Could you check a few things on this model? Use its own coordinates, in mm. Face numbers are marked on the shaded views. A direction names the side the tool comes from. Coordinates: 2 decimals unless noted, no trailing zeros. Order: outer loops, then holes, each group sorted by start corner. A loop starts at its lowest first (then second) coordinate and runs counter-clockwise, first axis right, second up. Notation, with made-up numbers: (14, 52.25) - (70, 52.25) arc R30 cw to (70, 76.25) - close; hole circle Ø2 at (77, -12). An arc over 180 degrees is marked (long way). Answer as a JSON object with one key per item and string values. Group by question number.
(1) Imagine slicing it at D-D, the plane x = 0. Write out the boundary of the cut face in (y, z).
(2) Please list where these lines run through material, in increasing order: probe 1 along Y at (x, z) = (0.75, -2); probe 2 along X at (y, z) = (-3.5, 0); probe 3 along Y at (x, z) = (9, 1.5).
(3) Which directions (+Z, -Z, +X, -X, +Y, -Y) give clear straight access to the entire face, cutting with the end or side of a thin tool? Please do the marked faces 1 and 2.
(4) Imagine slicing it at B-B, the plane x = -2.75. Write out the boundary of the cut face in (y, z).
(5) Imagine slicing it at A-A, the plane y = 1. Write out the boundary of the cut face in (x, z).
(6) Imagine slicing it at C-C, the plane z = -0.25. Write out the boundary of the cut face in (x, y).
(7) Will these pins go through, and if not, where does the flat tip stop? P1, Ø4, axis at y = -3.5, z = 2, coming from the +X side; P2, Ø2, axis at y = -2, z = 3, coming from the +X side; P3, Ø1.4, axis at x = 0, z = 0, coming from the +Y side.
(8) We'd pull the mould along Z, two halves only. Please class the marked faces 3, 4 and 5: pulls with the +Z half, pulls with the -Z half, needs draft (parallel to the pull), parting line crosses it, or undercut.
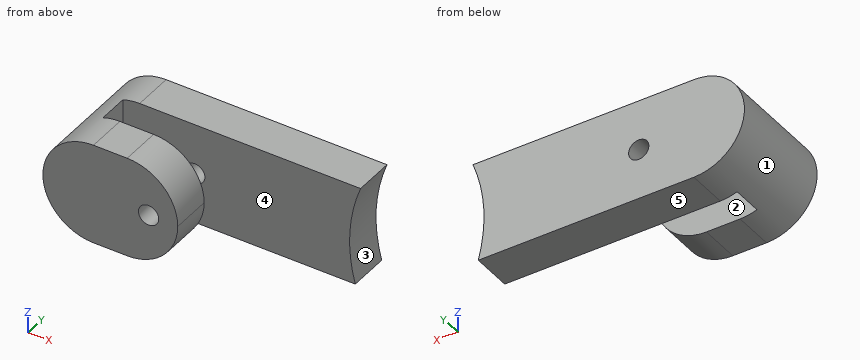
from build123d import *

# Parameters (mm, degrees)
SKETCH1_W           = 18.396209947
SKETCH1_H           = 7.5
BOSS_EXTRUDE1_DEPTH = 3
SKETCH3_W           = 7.837448939
SKETCH3_H           = 7.5
BOSS_EXTRUDE2_DEPTH = 3
SKETCH4_R           = 12
CUT_EXTRUDE2_DEPTH  = 3
SKETCH6_W           = 2.5
SKETCH6_H           = 7.5
BOSS_EXTRUDE3_DEPTH = 5.25
SKETCH7_W           = 7.5
SKETCH7_H           = 3
BOSS_EXTRUDE4_DEPTH = 7.5
CUT_EXTRUDE1_REACH  = 17.271
SKETCH2_R           = 0.75
FILLET1_R           = 3.75


with BuildPart() as part:
    # Sketch1 → Boss-Extrude1 (new body)
    with BuildSketch(Plane(origin=(0, 0, 0), x_dir=(1, 0, 0), z_dir=(0, 1, 0))):
        with Locations((9.198104974, 0)):
            Rectangle(SKETCH1_W, SKETCH1_H)
    extrude(amount=BOSS_EXTRUDE1_DEPTH)

    # Sketch3 → Boss-Extrude2 (add)
    with BuildSketch(Plane(origin=(0, 3, 0), x_dir=(1, 0, 0), z_dir=(0, 1, 0))):
        with Locations((-3.91872447, 0)):
            Rectangle(SKETCH3_W, SKETCH3_H)
    extrude(amount=-BOSS_EXTRUDE2_DEPTH)

    # Sketch4 → Cut-Extrude2 (cut)
    with BuildSketch(Plane(origin=(0, 3, 0), x_dir=(1, 0, 0), z_dir=(0, 1, 0))):
        with Locations((23.476391496, 0.596984019)):
            Circle(SKETCH4_R)
    extrude(amount=-CUT_EXTRUDE2_DEPTH, mode=Mode.SUBTRACT)

    # Sketch6 → Boss-Extrude3 (add)
    with BuildSketch(Plane.XZ):
        with Locations((-6.587448939, 0)):
            Rectangle(SKETCH6_W, SKETCH6_H)
    extrude(amount=BOSS_EXTRUDE3_DEPTH)

    # Sketch7 → Boss-Extrude4 (add)
    with BuildSketch(Plane(origin=(-5.337448939, 0, 0), x_dir=(0, 0, -1), z_dir=(1, 0, 0))):
        with Locations((0, -3.75)):
            Rectangle(SKETCH7_W, SKETCH7_H)
    extrude(amount=BOSS_EXTRUDE4_DEPTH)

    # Cut-Extrude1: up to this face of the body (flat: up to its plane)
    cut_extrude1_end = Plane(part.part.faces().sort_by_distance((-2.837448939, -5.25, 0))[0])
    # Sketch2 → Cut-Extrude1 (cut, up to the picked face)
    with BuildSketch(Plane(origin=(0, 3, 0), x_dir=(1, 0, 0), z_dir=(0, 1, 0)), mode=Mode.PRIVATE) as cut_extrude1_sk1:
        with Locations(Location((0, 0, 0), (0, 0, 90))):
            Circle(SKETCH2_R)
    cut_extrude1_tool1 = split(extrude(cut_extrude1_sk1.sketch, amount=-CUT_EXTRUDE1_REACH, mode=Mode.PRIVATE), bisect_by=cut_extrude1_end, keep=Keep.BOTH, mode=Mode.PRIVATE)
    add(cut_extrude1_tool1.solids().sort_by(Axis((0, 3, 0), (0, -1, 0)))[0], mode=Mode.SUBTRACT)

    # Fillet1
    # the kernel refuses this fillet: 3.75 mm, written as the material it takes off along each edge
    with BuildSketch(Plane(origin=(2.162551061, -14.625, -3.75), x_dir=(0, 0, 1), z_dir=(0, 1, 0))) as fillet1_piece_1:
        with BuildLine():
            CenterArc((FILLET1_R, -FILLET1_R), FILLET1_R, 90, 90)
            Line((0, -FILLET1_R), (0, 0))
            Line((0, 0), (FILLET1_R, 0))
        make_face()
    extrude(amount=12.375, mode=Mode.SUBTRACT)
    with BuildSketch(Plane(origin=(2.162551061, -2.25, 3.75), x_dir=(-1, 0, 0), z_dir=(0, -1, 0))) as fillet1_piece_2:
        with BuildLine():
            CenterArc((FILLET1_R, FILLET1_R), FILLET1_R, 180, 90)
            Line((0, FILLET1_R), (0, 0))
            Line((0, 0), (FILLET1_R, 0))
        make_face()
    extrude(amount=12.375, mode=Mode.SUBTRACT)
    with BuildSketch(Plane(origin=(-7.837448939, 12.375, 3.75), x_dir=(1, 0, 0), z_dir=(0, -1, 0)), Plane(origin=(-7.837448939, 12.375, -3.75), x_dir=(0, 0, 1), z_dir=(0, -1, 0))) as fillet1_piece_3:
        with BuildLine():
            CenterArc((FILLET1_R, -FILLET1_R), FILLET1_R, 90, 90)
            Line((0, -FILLET1_R), (0, 0))
            Line((0, 0), (FILLET1_R, 0))
        make_face()
    extrude(amount=27, mode=Mode.SUBTRACT)


solid = part.part
Result set:
{
 "1": {"outline": "(-5.25, -3.4) - (-2.25, -3.4) - (-2.25, -0.75) - (-5.25, -0.75) - close; (-5.25, 0.75) - (-2.25, 0.75) - (-2.25, 3.4) - (-5.25, 3.4) - close; (0, -3.75) - (3, -3.75) - (3, -0.75) - (0, -0.75) - close; (0, 0.75) - (3, 0.75) - (3, 3.75) - (0, 3.75) - close"},
 "2": {"probe 1": "y = -5.25 to -2.25, 0 to 3", "probe 2": "x = -7.84 to -0.75, 0.75 to 2.16", "probe 3": "y = 0 to 3"},
 "3": {"face 1": "-X, +Y, -Y", "face 2": "+Z, -Z, +X"},
 "4": {"outline": "(-5.25, -3.75) - (-2.25, -3.75) - (-2.25, 3.75) - (-5.25, 3.75) - close; (0, -3.75) - (3, -3.75) - (3, 3.75) - (0, 3.75) - close"},
 "5": {"outline": "(-4.09, -3.75) - (11.9, -3.75) arc R12 cw to (12.29, 3.75) - (-4.09, 3.75) arc R3.75 ccw to start; hole circle Ø1.5 at (0, 0)"},
 "6": {"outline": "(-7.83, -5.25) - (-0.71, -5.25) - (-0.71, -2.25) - (-5.34, -2.25) - (-5.34, 0) - (-0.71, 0) - (-0.71, 3) - (-7.83, 3) - close; (0.71, -5.25) - (2.15, -5.25) - (2.15, -2.25) - (0.71, -2.25) - close; (0.71, 0) - (11.48, 0) - (11.48, 3) - (0.71, 3) - close"},
 "7": {"P1": "stops at x = 2.16", "P2": "stops at x = 1.56", "P3": "passes through"},
 "8": {"face 3": "undercut", "face 4": "needs draft", "face 5": "pulls with the -Z half"}
}
